Read the model definition and answer for the solid it produces. Units are mm, in the model's axes. A direction names the side the tool comes from. Give positions to 0.01 mm unless a question says otherwise; leave off trailing zeros. Order: outer loops, then holes, each group sorted by start corner. A loop starts at its lowest first (then second) coordinate and runs counter-clockwise, first axis right, second up. Notation, with made-up numbers: (-14, 89.25) - (40, 89.25) arc R24 cw to (40, 125.25) - close; hole circle Ø7 at (74, 83.25). An arc over 180 degrees is marked (long way). Return JSON: item names as keys, results as strings.
Autodesk Inventor part; units mm, degrees
ref_plane "YZ Plane" through (0, 0, 0) normal (1, 0, 0) x (0, 1, 0)
ref_plane "XZ Plane" through (0, 0, 0) normal (0, 1, 0) x (-1, 0, 0)
ref_plane "XY Plane" through (0, 0, 0) normal (0, 0, 1) x (1, 0, 0)
sketch "Sketch1" plane through (0, 0, 0) normal (0, 1, 0) x (-1, 0, 0)
  circle A0 centre (0, 0) radius 1.175
  dimension "d0" = 2.35
extrude "Extrusion1" add sketch "Sketch1" along normal blind 8
sketch "Sketch2" plane through (0, 8, 0) normal (0, 1, 0) x (1, 0, 0)
  circle A0 centre (0, 0) radius 1.175
  circle A1 centre (0, 0) radius 1.925
  dimension "d3" = 3.85
extrude "Extrusion2" add sketch "Sketch2" along normal blind 2 contours A0 | A1
sketch "Sketch3" plane through (0, 10, 0) normal (0, 1, 0) x (1, 0, 0)
  line L0 (-0.4961, 0.7099) -> (0.3667, 0.7845)
  line L1 (0.3667, 0.7845) -> (0.8628, 0.0747)
  line L2 (0.8628, 0.0747) -> (0.4961, -0.7099)
  line L3 (0.4961, -0.7099) -> (-0.3667, -0.7845)
  line L4 (-0.3667, -0.7845) -> (-0.8628, -0.0747)
  line L5 (-0.8628, -0.0747) -> (-0.4961, 0.7099)
  point P0 (0, 0)
  point P1 (0, 0)
  dimension "d6" = 1.5
extrude "Extrusion3" cut sketch "Sketch3" against normal blind 1
equation "\"d0\" = M2_A"
equation "\"d3\" = M2_B"
properties part number "M2_SCREW_8MM"
Q1. A cutting plane is placed at A-A (z = 0.95). Write down the section's boundary in (x, y).
Values:
{"outline": "(-1.67, 8) - (-0.69, 8) - (-0.69, 0) - (0.69, 0) - (0.69, 8) - (1.67, 8) - (1.67, 10) - (-1.67, 10) - close"}
Q2. A cutting plane is placed at C-C (y = 6.75). Write down the section's boundary in (x, z) (3 decimals).
Values:
{"outline": "circle Ø2.35 at (0, 0)"}
Q3. A cutting plane is placed at D-D (y = 8.25). Write down the section's boundary in (x, z) (3 decimals), and give its area (3 significant figures).
Values:
{"outline": "circle Ø3.85 at (0, 0)", "area": "11.6 mm²"}
Q4. Determine the mould class of faces 4 (the flat face through (0, 10, 1)), 5 (the flat face through (0.071, 9.507, 0.747)), 6 (the cylindrical face through (-0.42, 8.99, -1.88)) for opening direction X: released by +X, released by -X, zero draft, split by the parting line, or undercut.
Values:
{"face 4": "zero draft", "face 5": "undercut", "face 6": "split by the parting line"}
Q5. For faces 1 (the flat face through (0, 9, 0)), 2 (the flat face through (0, 0, 0)), 3 (the flat face through (1, 8, -1)), determine the directions among +Z, -Z, +X, -X, +Y, -Y from which every point of the face is accessible in a straight line to the end or side of a thin tool.
Values:
{"face 1": "+Y", "face 2": "+Z, -Z, +X, -X, -Y", "face 3": "-Y"}
Q6. A cutting plane is placed at B-B (x = 0). Write down the section's boundary in (y, z) (3 decimals), and give its area (3 significant figures).
Values:
{"outline": "(0, -1.175) - (8, -1.175) - (8, -1.925) - (10, -1.925) - (10, -0.753) - (9, -0.753) - (9, 0.753) - (10, 0.753) - (10, 1.925) - (8, 1.925) - (8, 1.175) - (0, 1.175) - close", "area": "25.0 mm²"}
Q7. Consider L1, parallel to Y at x = -0.15, z = 0.4; L2, parallel to Y at x = -0.2, z = -1.3; L3, parallel to Z at x = 0.6, y = 9.25. Determine where each line is inside the solid, lowest interval first.
Values:
{"L1": "y = 0 to 9", "L2": "y = 8 to 10", "L3": "z = -1.83 to -0.45, 0.49 to 1.83"}
Q8. Given pin 1 (2 mm diameter, centred on x = 0, y = 3.5, fed in from -Z) (3 decimals); pin 2 (1 mm diameter, centred on x = -1, y = 3.5, fed in from -Z), each flat-ended and moving along its own axis, determine where each tip first touches the part or whether it passes through.
Values:
{"pin 1": "stops at z = -1.175", "pin 2": "stops at z = -1.06"}
